from build123d import *

# Parameters (mm, degrees)
F1_DEPTH = 2
F2_COUNT = 10


with BuildPart() as f1:
    # F0 (on Top) → F1 (new body)
    with BuildSketch(Plane.XY):
        with BuildLine():
            ThreePointArc((0, 7.6807912749), (-5.4311395954, -5.4311395954), (7.6807912749, 0))
            ThreePointArc((7.6807912749, 0), (6.1208653438, 4.6399959108), (2.0747120882, 7.3952771659))
            Line((2.0747120882, 7.3952771659), (0, 0))
            Line((0, 0), (0, 7.6807912749))
        make_face()
        with BuildLine():
            Line((0, 0), (2.0747120882, 7.3952771659))
            ThreePointArc((2.0747120882, 7.3952771659), (1.0471328182, 7.6090779645), (0, 7.6807912749))
            Line((0, 7.6807912749), (0, 0))
        make_face()
        with BuildLine():
            ThreePointArc((0, 7.6807912749), (1.0471328182, 7.6090779645), (2.0747120882, 7.3952771659))
            Line((2.0747120882, 7.3952771659), (2.7417573147, 9.7729489207))
            Line((2.7417573147, 9.7729489207), (0, 9.7729489207))
            Line((0, 9.7729489207), (0, 7.6807912749))
        make_face()
    extrude(amount=F1_DEPTH)

    # F2: F1 ×10 about axis
    f2_axis = Axis((0, 0, 0), (0, 0, -1))


with BuildPart() as f1_1:
    add(f1.part)
    for i in range(1, F2_COUNT):
        add(f1.part.rotate(f2_axis, i * 360 / F2_COUNT))


solid = f1_1.part
Design review of the part built by this model. Coordinates are the model's own, in mm. A direction names the side the tool comes from. Give positions to 0.01 mm unless a question says otherwise; leave off trailing zeros. Loops run counter-clockwise (first coordinate to the right, second up) from the corner with the lowest first, then second, coordinate; pieces in that order, holes last. Notation, with made-up numbers: M -8,-24 L 43,-24 A20 cw 43,-15 Z; hole C 32,61 d2. An arc over 180 degrees is marked long. One line per question, with ' | ' between items. Start each with the question number.
1. The part is to be moulded in two halves that separate along Y. For faces 6 (the face through (8.865, -4.342, 0.986)), 7 (the face through (-6.98, -5.52, 0.99)), 8 (the face through (5.138, 7.072, 0.986)), say which applies: released by +Y, released by -Y, zero draft, split by the parting line, or undercut.
2. Insertion check: P1, Ø0.6, axis at y = 9, z = 1.5, coming from the -X side. The pin has a flat end and moves straight along its axis. Give the tip position at first contact, or say it passes through.
3. Add section D-D (x = -4.25). Write out the cut boundary in (y, z), plus the area to 3 significant figures.
4. Add section C-C (y = 5). Write out the cut boundary in (x, z), plus the area to 3 significant figures.
5. For faces 1 (the face through (6.98, 5.52, 0.99)), 2 (the face through (9.724, 1.698, 0.986)), 3 (the face through (-8.31, 2.7, 0.99)), 4 (the face through (3.09, -8.34, 0.99)), 5 (the face through (-7.405, 4.933, 0.986)), list the 3-axis set-ups (+Z, -Z, +X, -X, +Y, -Y) from which the entire face can be reached by the end or side of a thin tool; tool diameter is ignored.
6. Add section B-B (x = 4). Write out the cut boundary in (y, z).
7. To check wall thickness, follow L1, parallel to X at y = 0, z = 1.1; L2, parallel to X at y = 7, z = 0.55; L3, parallel to Y at x = 5, z = 1. State the ranges of each line that lie inside material, in increasing order.
8. Add section A-A (y = -8.25). Write out the cut boundary in (x, z).
Worked out:
1) face 6: released by -Y | face 7: undercut | face 8: released by +Y
2) P1: stops at x = -4.65
3) outline: M -6.4,0 L 8.99,0 L 8.99,2 L -6.4,2 Z | area: 30.8 mm²
4) outline: M -8.65,0 L -7.51,0 L -7.51,2 L -8.65,2 Z; M -5.83,0 L 6.32,0 L 6.32,2 L -5.83,2 Z | area: 26.6 mm²
5) face 1: +Z, -Z, +X | face 2: +Z, -Z, +X, +Y | face 3: +Z, -Z, -X | face 4: +Z, -Z, -Y | face 5: +Z, -Z, +Y
6) outline: M -9.17,0 L 6.56,0 L 6.56,2 L -9.17,2 Z
7) L1: x = -7.68 to 7.68 | L2: x = -5.09 to 3.16, 5.09 to 6.99 | L3: y = -8.45 to -6.88, -5.83 to 6.88
8) outline: M -2.31,0 L 0,0 L 0,2 L -2.31,2 Z; M 3.06,0 L 5.27,0 L 5.27,2 L 3.06,2 Z
